```python
from build123d import *

# Parameters (mm, degrees)
F0_W      = 152.4
F0_H      = 127
F1_DEPTH  = 76.2
F2_W      = 27.119612
F2_H      = 50.8
F3_DEPTH  = 76.201
F4_R      = 19.05
F5_DEPTH  = 25.4
F7_DEPTH  = 25.4
F3_FACE_W = 16.120646
F3_FACE_H = 76.2
F9_DEPTH  = 38.1
F8_R      = 7.927826
F10_DEPTH = 40.64


with BuildPart() as f1:
    # F0 (on Front) → F1 (new body)
    with BuildSketch(Plane.XZ):
        Rectangle(F0_W, F0_H)
    extrude(amount=F1_DEPTH)

    # F2 (on face) → F3 (cut, through all)
    with BuildSketch(Plane.XZ.offset(76.2)):
        with Locations((-62.640194, 38.1)):
            Rectangle(F2_W, F2_H)
        Polygon((76.2, 63.5), (27.119612, 63.5), (27.119612, -38.1), (42.236097, -38.1), (42.236097, 0), (58.356743, 0), (58.356743, -38.1), (76.2, -38.1), align=None)
    extrude(amount=-F3_DEPTH, mode=Mode.SUBTRACT)

    # F4 (on face) → F5 (join)
    with BuildSketch(Plane.XZ.offset(76.2)):
        with Locations((-32.980844, -63.5)):
            Circle(F4_R)
        with Locations((55.411834, -63.5)):
            Circle(F4_R)
    extrude(amount=F5_DEPTH)

    # F6 (on face) → F7 (join)
    with BuildSketch(Plane(origin=(0, 0, 0), x_dir=(-1, 0, 0), z_dir=(0, 1, 0))):
        with BuildLine():
            Line((51.936118, -63.5), (13.836118, -63.5))
            ThreePointArc((13.836118, -63.5), (32.886118, -82.55), (51.936118, -63.5))
        make_face()
        with BuildLine():
            ThreePointArc((-75.149854, -63.5), (-56.099854, -82.55), (-37.049854, -63.5))
            Line((-37.049854, -63.5), (-75.149854, -63.5))
        make_face()
        with BuildLine():
            ThreePointArc((51.936118, -63.5), (32.886118, -44.45), (13.836118, -63.5))
            Line((13.836118, -63.5), (51.936118, -63.5))
        make_face()
        with BuildLine():
            Line((-75.149854, -63.5), (-37.049854, -63.5))
            ThreePointArc((-37.049854, -63.5), (-56.099854, -44.45), (-75.149854, -63.5))
        make_face()
    extrude(amount=F7_DEPTH)

    # F3_face (on face) → F9 (cut)
    with BuildSketch(Plane(origin=(50.29642, -38.1, 0), x_dir=(1, 0, 0), z_dir=(0, 0, 1))):
        Rectangle(F3_FACE_W, F3_FACE_H)
    extrude(amount=-F9_DEPTH, mode=Mode.SUBTRACT)

    # F8 (on Top) → F10 (join)
    with BuildSketch(Plane.XY):
        with Locations((50.55435, -39.241035)):
            Circle(F8_R)
    extrude(amount=-F10_DEPTH)


solid = f1.part
```
Geometry: final body of the model. Coordinates: model frame, mm. A direction names the side the tool comes from. Coordinates: 2 decimals unless noted, no trailing zeros. Order: outer loops, then holes, each group sorted by start corner. A loop starts at its lowest first (then second) coordinate and runs counter-clockwise, first axis right, second up. Notation, with made-up numbers: (-35, 54.25) -> (-15, 54.25) arc R12 cw to (-15, 69.25) -> close; hole circle Ø4 at (82, 86). An arc over 180 degrees is marked (long way). Write item = value, one per line.
(1) Pull-direction query (X, two-part tool) for faces 1 (the flat face through (76.2, -38, -51)), 2 (the cylindrical face through (-37.1, -88.7, -82.1)), 3 (the flat face through (-33, 25.4, -63)); classes: pulls with the +X half, pulls with the -X half, needs draft (parallel to the pull), parting line crosses it, or undercut.
Solved:
face_1 = pulls with the +X half
face_2 = undercut
face_3 = needs draft
(2) Access query for faces 4 (the flat face through (56, 0, -71)), 5 (the flat face through (-63, -39, 12.7)), 6 (the cylindrical face through (-17.769, 12.522, -75.092)), 7 (the cylindrical face through (51.3, -88.7, -82.1)), 8 (the cylindrical face through (42.634, -38.892, -18.783)). Directions: +Z, -Z, +X, -X, +Y, -Y. A direction counts if a zero-diameter tool reaches every point of the face in a straight line with its end or side. Return the directions, or none.
Solved:
face_4 = -Z, +X, -X
face_5 = +Z, -X, +Y, -Y
face_6 = +Y
face_7 = -Y
face_8 = +Z
(3) Cut plane C-C on x = -17.5. Return loops of the section in (y, z), plus the area to 3 significant figures.
Solved:
outline = (-101.6, -74.6) -> (-76.2, -74.6) -> (-76.2, -63.5) -> (0, -63.5) -> (0, -74.73) -> (25.4, -74.73) -> (25.4, -52.27) -> (0, -52.27) -> (0, 63.5) -> (-76.2, 63.5) -> (-76.2, -52.4) -> (-101.6, -52.4) -> close
area = 10,800 mm²
(4) Pin query (flat end, axial travel): pin 1 Ø6 at (x, y) = (59, -33.5) entering from -Z; pin 2 Ø24.5 at (x, y) = (48, -42.5) entering from +Z; pin 3 Ø1.5 at (y, z) = (-33, 8) entering from +X. Return the tip coordinate at first contact, or that it passes through.
Solved:
pin_1 = -63.5
pin_2 = 0
pin_3 = 27.12
(5) Cut plane D-D on z = 48. Return loops of the section in (x, y).
Solved:
outline = (-49.08, -76.2) -> (27.12, -76.2) -> (27.12, 0) -> (-49.08, 0) -> close
(6) Cut plane B-B on y = -9. Return loops of the section in (x, z).
Solved:
outline = (-76.2, -63.5) -> (76.2, -63.5) -> (76.2, -38.1) -> (27.12, -38.1) -> (27.12, 63.5) -> (-49.08, 63.5) -> (-49.08, 12.7) -> (-76.2, 12.7) -> close
(7) Line query: line 1 (X direction, y = 16.5, z = -63); line 2 (X direction, y = -74, z = -4.5); line 3 (Z direction, x = -56.5, y = -75). Output: solid intervals per line, ascending.
Solved:
line_1 = -51.93 to -13.84, 37.06 to 75.14
line_2 = -76.2 to 27.12
line_3 = -63.5 to 12.7
(8) Cut plane A-A on z = -18. Return loops of the section in (x, y), plus the area to 3 significant figures.
Solved:
outline = (-76.2, -76.2) -> (27.12, -76.2) -> (27.12, 0) -> (-76.2, 0) -> close; circle Ø15.86 at (50.55, -39.24)
area = 8,070 mm²
